```python
from build123d import *

# Parameters (mm, degrees)
F0_R     = 10
F0_R_2   = 5
F0_R_3   = 2.5
F1_DEPTH = 3
F2_DEPTH = 10


with BuildPart() as f1:
    # F0 (on Top) → F1 (new body)
    with BuildSketch(Plane.XY):
        with BuildLine():
            Line((2.605609, -11.713701), (35.035962, -4.499856))
            ThreePointArc((35.035962, -4.499856), (39.477433, -0.450106), (35.930912, 4.402659))
            Line((35.930912, 4.402659), (4.857465, 10.972923))
            ThreePointArc((4.857465, 10.972923), (-11.941319, 1.185285), (2.605609, -11.713701))
        make_face()
        Circle(F0_R, mode=Mode.SUBTRACT)
        with Locations((20, 0)):
            Circle(F0_R_2, mode=Mode.SUBTRACT)
        with Locations((35, 0)):
            Circle(F0_R_3, mode=Mode.SUBTRACT)
        Circle(F0_R)
        with Locations((20, 0)):
            Circle(F0_R_2)
        with Locations((35, 0)):
            Circle(F0_R_3)
    extrude(amount=F1_DEPTH)

    # F0 (on Top) → F2 (join)
    with BuildSketch(Plane.XY):
        Circle(F0_R)
        with Locations((20, 0)):
            Circle(F0_R_2)
        with Locations((35, 0)):
            Circle(F0_R_3)
    extrude(amount=F2_DEPTH)


solid = f1.part
```
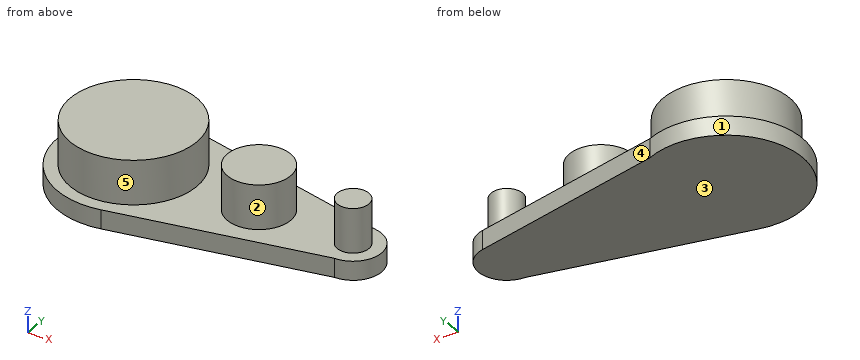
Verification items for the finished model (mm, model axes). Face numbers are marked on the shaded views. A direction names the side the tool comes from. Give positions to 0.01 mm unless a question says otherwise; leave off trailing zeros. Order: outer loops, then holes, each group sorted by start corner. A loop starts at its lowest first (then second) coordinate and runs counter-clockwise, first axis right, second up. Notation, with made-up numbers: M -27.75,5.5 L 23.25,5.5 A29 cw 23.25,37.5 Z; hole C -11,-7 d3. An arc over 180 degrees is marked long. Answer in a Markdown table with one row per item. Add a question column.
Item 1: Section check D-D, the plane z = 1.25. Enter the section's corners in (x, y).
Item 2: Mould release check, pull along X, two halves, no side actions. Record for the marked faces 1, 2 and 3: released by +X, released by -X, zero draft, split by the parting line, or undercut.
Item 3: Section check B-B, the plane y = 0. Enter the section's corners in (x, z).
Item 4: Tool access check on the marked faces 4 and 5. Record the directions out of +Z, -Z, +X, -X, +Y, -Y that give a thin tool (end or side, any length) a straight path to the whole face; none if there is none.
Item 5: Section check A-A, the plane x = 0. Enter the section's corners in (y, z).
Item 6: Scan lines: probe 1 along X at (y, z) = (-2.25, 5); probe 2 along X at (y, z) = (4, 7); probe 3 along X at (y, z) = (0.25, 6.75). Record each from-to range of solid material in increasing order. Write a range as from..to.
Item 7: Section check C-C, the plane z = 7.5. Enter the section's corners in (x, y), and give its area (3 significant figures).
Item 8: Gauge pin test, flat ends, axial feed: pin 1 (6 mm diameter, centred on x = 13, z = 8, fed in from -Y); pin 2 (1.5 mm diameter, centred on x = -2, z = 2.5, fed in from -Y); pin 3 (1.5 mm diameter, centred on x = 3.5, z = 4, fed in from -Y). Record the tip position at first contact, or that the pin passes through.
Filled sheet:
| question | item | result |
|---|---|---|
| 1 | outline | M 2.61,-11.71 L 35.04,-4.5 A4.5 ccw 35.93,4.4 L 4.86,10.97 A12 ccw long Z |
| 2 | face 1 | split by the parting line |
| 2 | face 2 | undercut |
| 2 | face 3 | zero draft |
| 3 | outline | M -12,0 L 39.5,0 L 39.5,3 L 37.5,3 L 37.5,10 L 32.5,10 L 32.5,3 L 25,3 L 25,10 L 15,10 L 15,3 L 10,3 L 10,10 L -10,10 L -10,3 L -12,3 Z |
| 4 | face 4 | +Z, -Z, +X, +Y |
| 4 | face 5 | +Z |
| 5 | outline | M -12,0 L 12,0 L 12,3 L 10,3 L 10,10 L -10,10 L -10,3 L -12,3 Z |
| 6 | probe 1 | x = -9.74..9.74, 15.53..24.47, 33.91..36.09 |
| 6 | probe 2 | x = -9.17..9.17, 17..23 |
| 6 | probe 3 | x = -10..10, 15.01..24.99, 32.51..37.49 |
| 7 | outline | C 0,0 d20; C 20,0 d10; C 35,0 d5 |
| 7 | area | 412 mm^2 |
| 8 | pin 1 | stops at y = -3 |
| 8 | pin 2 | stops at y = -11.93 |
| 8 | pin 3 | stops at y = -9.61 |
